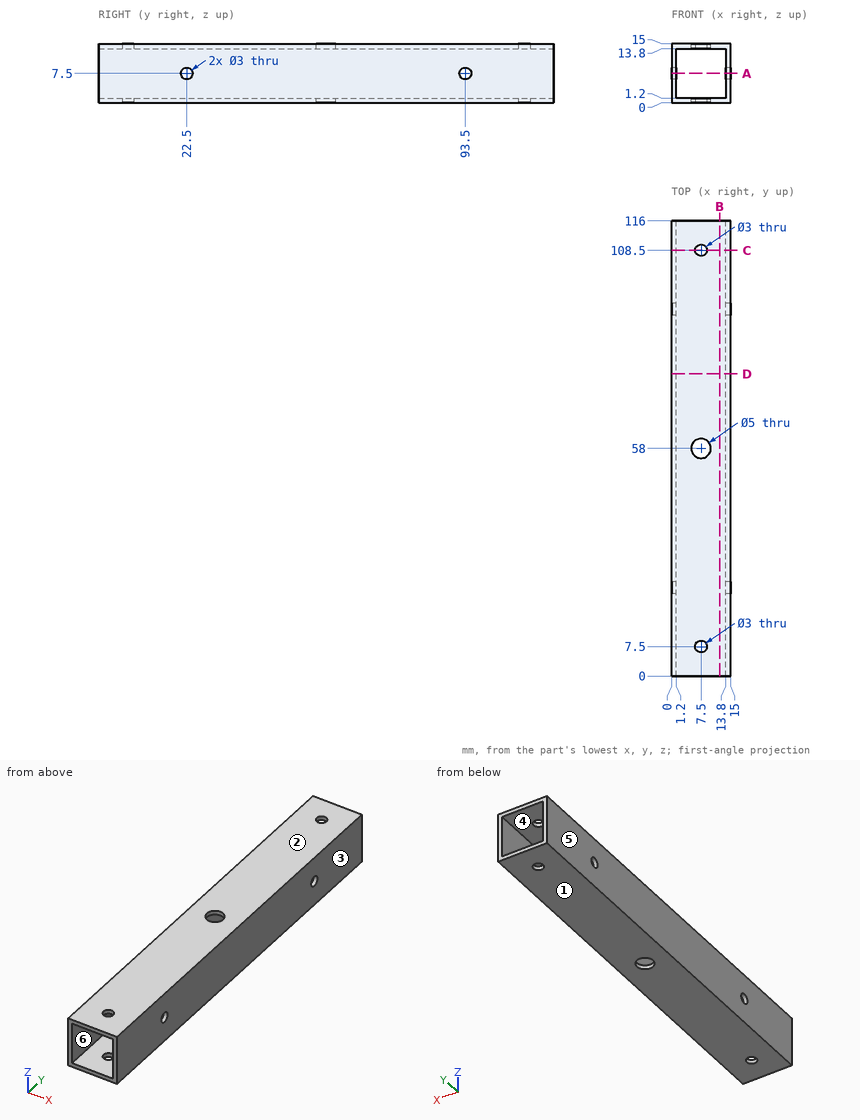
Source: three-view drawing plus pictorial views. Frame: mm from the lowest corner of the part. A direction names the side the tool comes from. Give positions to 0.01 mm unless a question says otherwise; leave off trailing zeros. Loops run counter-clockwise (first coordinate to the right, second up) from the corner with the lowest first, then second, coordinate; pieces in that order, holes last. Notation, with made-up numbers: (83.25, -18.75) -> (135.25, -18.75) arc R34 ccw to (135.25, 15.25) -> close; hole circle Ø5 at (6, -22). An arc over 180 degrees is marked (long way). Use a Markdown table: item, result. Add a question column.
(1) Section query A-A (z = 7.5). Output: boundary loops of the cut face in (x, y), then the cut area to 3 significant figures.
(2) Ray query, line 1 (Y direction, x = 0.5, z = 7.5); line 2 (Z direction, x = 7.25, y = 44); line 3 (Z direction, x = 0.35, y = 22.5). Return the intervals inside material, ascending.
(3) Section query C-C (y = 108.5). Output: boundary loops of the cut face in (x, z).
(4) Access query for the marked faces 5 and 6. Directions: +Z, -Z, +X, -X, +Y, -Y. A direction counts if a zero-diameter tool reaches every point of the face in a straight line with its end or side. Return the directions, or none.
(5) Section query B-B (x = 12.25). Output: boundary loops of the cut face in (y, z), then the cut area to 3 significant figures.
(6) Pull-direction query (Z, two-part tool) for the marked faces 1, 2, 3 and 4; classes: +Z half, -Z half, draft (parallel to the pull), parting line (faces both ways), or undercut.
(7) First-contact query: pin 1 Ø2.5 at (x, y) = (7.5, 7.5) entering from -Z. Flat tip, straight axial feed; report the tip coordinate or a pass-through.
(8) Section query D-D (y = 77). Output: boundary loops of the cut face in (x, z), then the cut area to 3 significant figures.
Checked values:
| question | item | result |
|---|---|---|
| 1 | outline | (0, 0) -> (1.2, 0) -> (1.2, 21) -> (0, 21) -> close; (0, 24) -> (1.2, 24) -> (1.2, 92) -> (0, 92) -> close; (0, 95) -> (1.2, 95) -> (1.2, 116) -> (0, 116) -> close; (13.8, 0) -> (15, 0) -> (15, 21) -> (13.8, 21) -> close; (13.8, 24) -> (15, 24) -> (15, 92) -> (13.8, 92) -> close; (13.8, 95) -> (15, 95) -> (15, 116) -> (13.8, 116) -> close |
| 1 | area | 264 mm^2 |
| 2 | line 1 | 0 to 21, 24 to 92, 95 to 116 |
| 2 | line 2 | 0 to 1.2, 13.8 to 15 |
| 2 | line 3 | 0 to 6, 9 to 15 |
| 3 | outline | (0, 0) -> (6, 0) -> (6, 1.2) -> (1.2, 1.2) -> (1.2, 13.8) -> (6, 13.8) -> (6, 15) -> (0, 15) -> close; (9, 0) -> (15, 0) -> (15, 15) -> (9, 15) -> (9, 13.8) -> (13.8, 13.8) -> (13.8, 1.2) -> (9, 1.2) -> close |
| 4 | face 5 | +Z, -Z, -X, +Y, -Y |
| 4 | face 6 | +Y, -Y |
| 5 | outline | (0, 0) -> (116, 0) -> (116, 1.2) -> (0, 1.2) -> close; (0, 13.8) -> (116, 13.8) -> (116, 15) -> (0, 15) -> close |
| 5 | area | 278 mm^2 |
| 6 | face 1 | -Z half |
| 6 | face 2 | +Z half |
| 6 | face 3 | draft |
| 6 | face 4 | undercut |
| 7 | pin 1 | through |
| 8 | outline | (0, 0) -> (15, 0) -> (15, 15) -> (0, 15) -> close; hole (1.2, 1.2) -> (13.8, 1.2) -> (13.8, 13.8) -> (1.2, 13.8) -> close |
| 8 | area | 66.2 mm^2 |
